from build123d import *

# Parameters (mm, degrees)
RESSALTO_EXTRUS_O1_DEPTH   = 10
CORTE_EXTRUS_O1_DEPTH      = 112.394113732
CORTE_EXTRUS_O1_DEPTH_BACK = 112.394113732
ESBO_O2_R                  = 5
ESBO_O4_R                  = 10
RESSALTO_EXTRUS_O2_DEPTH   = 25


with BuildPart() as part:
    # Esboço1 → Ressalto-extrusão1 (new body)
    with BuildSketch(Plane.XY):
        with BuildLine():
            Line((-51.939383922, 71.964552472), (-51.939383922, -88.035447528))
            ThreePointArc((-51.939383922, -88.035447528), (-41.939383922, -98.035447528), (-31.939383922, -88.035447528))
            Line((-31.939383922, -88.035447528), (-31.939383922, 71.964552472))
            Line((-31.939383922, 71.964552472), (-51.939383922, 71.964552472))
        make_face()
    extrude(amount=RESSALTO_EXTRUS_O1_DEPTH)

    # Esboço2 → Corte-extrusão1 (cut, two sides: drawn at the far end of the back side and taken through both)
    with BuildSketch(Plane.XY.offset(10).offset(-CORTE_EXTRUS_O1_DEPTH_BACK)):
        with Locations((-41.939383922, -88.035447528)):
            Circle(ESBO_O2_R)
    extrude(amount=CORTE_EXTRUS_O1_DEPTH + CORTE_EXTRUS_O1_DEPTH_BACK, mode=Mode.SUBTRACT)

    # Esboço4 → Ressalto-extrusão2 (add)
    with BuildSketch(Plane.XY.offset(10)):
        with Locations((-41.939383922, 71.964552472)):
            Circle(ESBO_O4_R)
    extrude(amount=-RESSALTO_EXTRUS_O2_DEPTH)


solid = part.part
Build history of the part. All positions in model axes, mm. Give positions to 0.01 mm unless a question says otherwise; leave off trailing zeros. Order: outer loops, then holes, each group sorted by start corner. A loop starts at its lowest first (then second) coordinate and runs counter-clockwise, first axis right, second up. Notation, with made-up numbers: M 62.25,28.5 L 84.25,28.5 A5 cw 84.25,36.5 Z; hole C 31,40 d4. An arc over 180 degrees is marked long. Use one line per item in the form item = value.
Q1. Slice it at D-D, the plane z = -6.5. Write the cut outline in (x, y).
Conclusion:
outline = C -41.94,71.96 d20
Q2. Slice it at B-B, the plane x = -44. Write the cut outline in (y, z).
Conclusion:
outline = M -97.82,0 L -92.59,0 L -92.59,10 L -97.82,10 Z; M -83.48,0 L 62.18,0 L 62.18,-15 L 81.75,-15 L 81.75,10 L -83.48,10 Z
Q3. Slice it at C-C, the plane y = 15. Write the cut outline in (x, z), and give its area (3 significant figures).
Conclusion:
outline = M -51.94,0 L -31.94,0 L -31.94,10 L -51.94,10 Z
area = 200 mm2
Q4. Slice it at A-A, the plane z = 3.5. Write the cut outline in (x, y).
Conclusion:
outline = M -51.94,-88.04 A10 ccw -31.94,-88.04 L -31.94,71.96 A10 ccw -51.94,71.96 Z; hole C -41.94,-88.04 d10
Q5. Wall check: probe 1 along Z at (x, y) = (-41, -27.5); probe 2 along Y at (x, z) = (-44.25, 3.25); probe 3 along Y at (x, z) = (-37.5, 7.5). Give the ranges that are in metal, low to high.
Conclusion:
probe_1 = 0 to 10
probe_2 = -97.76 to -92.47, -83.6 to 81.69
probe_3 = -97 to -90.34, -85.74 to 80.93
Q6. Pin check, flat tips, straight feed: P1, Ø1, axis at x = -39.5, z = -11, coming from the -Y side; P2, Ø4, axis at x = -38, z = 4, coming from the -Y side; P3, Ø8, axis at x = -41.94, y = -88.04, coming from the +Z side; P4, Ø4, axis at x = -34, z = 0, coming from the -Y side. Stop position of each tip, or through.
Conclusion:
P1 = 62.15
P2 = -97.85
P3 = through
P4 = -96.08
Q7. Pull direction X, two halves, no side cores. Call faces 1 (the flat face through (-42, 72, -15)), 2 (the cylindrical face through (-43.24, 81.88, -5.1)), 3 (the cylindrical face through (-43.023, -92.917, 4.93)): released by +X, released by -X, zero draft, split by the parting line, or undercut.
Conclusion:
face_1 = zero draft
face_2 = split by the parting line
face_3 = undercut
